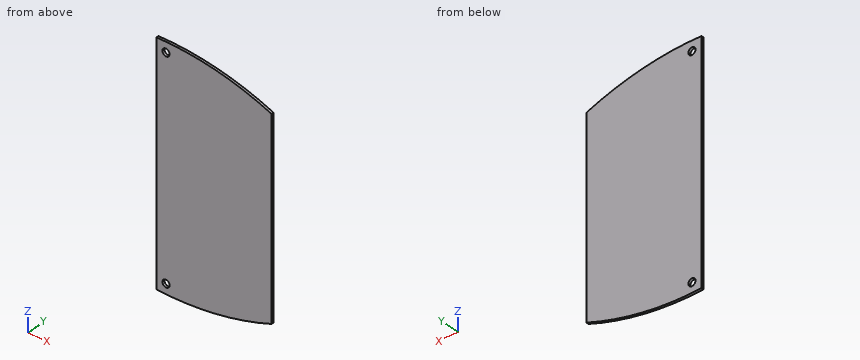
Autodesk Inventor part; units mm, degrees
ref_plane "YZ Plane" through (0, 0, 0) normal (1, 0, 0) x (0, 1, 0)
ref_plane "XZ Plane" through (0, 0, 0) normal (0, 1, 0) x (-1, 0, 0)
ref_plane "XY Plane" through (0, 0, 0) normal (0, 0, 1) x (1, 0, 0)
sketch "Sketch1" plane through (0, 0, 0) normal (0, 1, 0) x (-1, 0, 0)
  line L0 (76.2, -152.4) -> (76.2, 0)
  line L1 (0, 0) -> (0, -12.7)
  arc A0 (76.2, 0) -> (0, -12.7) centre (68.7675, -190.355) ccw
  line L2 (0, -152.4) -> (0, -139.7)
  arc A1 (0, -139.7) -> (76.2, -152.4) centre (68.7675, 37.955) ccw
  line L3 (0, -139.7) -> (0, -12.7)
  dimension "d0" = 152.4
  dimension "d1" = 76.2
  dimension "d17" = 12.7
  dimension "d18" = 190.5
  dimension "d20" = 190.5
extrude "Extrusion1" add sketch "Sketch1" along normal blind 1.5875
sketch "Sketch2" plane through (0, 1.5875, 0) normal (0, 1, 0) x (1, 0, 0)
  line L0 (-76.2, 0) -> (0, 0)
  line L1 (-76.2, 0) -> (-76.2, 12.7)
  line L2 (-76.2, 152.4) -> (-76.2, 0)
  line L3 (-76.2, 12.7) -> (-63.5, 0)
  line L4 (-63.5, 0) -> (-76.2, 0)
  line L5 (-76.2, 0) -> (-69.85, 6.35)
  line L6 (0, 0) -> (0, 12.7)
  line L7 (0, 0) -> (0, 152.4)
  line L8 (-76.2, 152.4) -> (-63.5, 152.4)
  line L9 (0, 152.4) -> (-76.2, 152.4)
  line L10 (-63.5, 152.4) -> (-76.2, 139.7)
  line L11 (-76.2, 139.7) -> (-76.2, 152.4)
  line L12 (-76.2, 152.4) -> (-69.85, 146.05)
  line L13 (-76.2, 152.4) -> (-67.2197, 152.4) construction
  dimension "d4" = 12.7
  dimension "d5" = 45
  dimension "d6" = 12.7
  dimension "d14" = 12.7
  dimension "d15" = 45
  dimension "d16" = 45
hole "Hole1" at (-69.85, 1.5875, -6.35) at (-69.85, 1.5875, -146.05) direction (0, -1, 0) diameter 4.7625 end through all
properties part number "shoot2" material "ABS Plastic"
Verification items for the finished model (mm, model axes). Coordinates: 2 decimals unless noted, no trailing zeros. Order: outer loops, then holes, each group sorted by start corner. A loop starts at its lowest first (then second) coordinate and runs counter-clockwise, first axis right, second up. Notation, with made-up numbers: (48, -17) -> (101, -17) arc R22 cw to (101, -4) -> close; hole circle Ø11 at (39, 71.25). An arc over 180 degrees is marked (long way). Answer as CSV lines item,"result". Start each with the question number.
1) Cross-section at D-D, the plane x = -30. Record the boundary of the cut face in (y, z).
2) Cross-section at C-C, the plane z = -6.35. Record the boundary of the cut face in (x, y), then the cut area to 3 significant figures.
3) Cross-section at B-B, the plane x = -69.85. Record the boundary of the cut face in (y, z), then the cut area to 3 significant figures.
4) Cross-section at A-A, the plane y = 0.95. Give the number of separate pieces and of enclosed holes in the cut face, then the cut area to 3 significant figures.
5) Material ranges on L1, parallel to Z at x = -69.85, y = 0.9; L2, parallel to Z at x = -29.5, y = 0.7; L3, parallel to Z at x = -64.5, y = 0.2, recorded low to high. Write a range as [from, to].
Conclusion:
1,outline,"(0, -148.56) -> (1.59, -148.56) -> (1.59, -3.84) -> (0, -3.84) -> close"
2,outline,"(-76.2, 0) -> (-72.23, 0) -> (-72.23, 1.59) -> (-76.2, 1.59) -> close; (-67.47, 0) -> (-19.45, 0) -> (-19.45, 1.59) -> (-67.47, 1.59) -> close"
2,area,"82.5 mm²"
3,outline,"(0, -152.54) -> (1.59, -152.54) -> (1.59, -148.43) -> (0, -148.43) -> close; (0, -143.67) -> (1.59, -143.67) -> (1.59, -8.73) -> (0, -8.73) -> close; (0, -3.97) -> (1.59, -3.97) -> (1.59, 0.14) -> (0, 0.14) -> close"
3,area,"227 mm²"
4,separate pieces,"1"
4,enclosed holes,"2"
4,area,"11,000 mm²"
5,L1,"z = [-152.54, -148.43], [-143.67, -8.73], [-3.97, 0.14]"
5,L2,"z = [-148.45, -3.95]"
5,L3,"z = [-152.5, 0.1]"
